Can you work these out from the drawing? Everything is in mm from the part's minimum corner. A direction names the side the tool comes from. Coordinates: 2 decimals unless noted, no trailing zeros. Order: outer loops, then holes, each group sorted by start corner. A loop starts at its lowest first (then second) coordinate and runs counter-clockwise, first axis right, second up. Notation, with made-up numbers: (28, -29) - (47, -29) arc R25 ccw to (47, 0) - close; hole circle Ø9 at (12, -6.75). An arc over 180 degrees is marked (long way). Use a Markdown table: item, result. Add a question column.
(1) I want a section at A-A (x = 3). List the corners of the cut face in (y, z) for me.
(2) For pin 1 Ø2 at (x, y) = (3, 2.2) entering from +Z; pin 2 Ø2.5 at (y, z) = (8.7, 4) entering from -X, each with a flat end and sliding along its axis, tell me the tip position at first contact or that it passes through.
(3) We'd pull the mould along Z, two halves only. Please class the marked faces 3, 4, 5 and 6: pulls with the +Z half, pulls with the -Z half, needs draft (parallel to the pull), parting line crosses it, or undercut.
(4) On a 3-axis mill with a long thin cutter (end or side, diameter ignored), from which of +Z, -Z, +X, -X, +Y, -Y can I reach the whole of each face in a straight line? I mean the marked faces 1 and 2. Say none if no direction works.
(5) I want a section at D-D (z = 6.75). List the corners of the cut face in (x, y) for me, and give its area (3 significant figures).
(6) I want a section at C-C (x = 0.9). List the corners of the cut face in (y, z) for me.
(7) If I drill on L1, parallel to Y at x = 3, z = 6.25; L2, parallel to Z at x = 1.9, y = 42.7; L3, parallel to Y at x = 3, z = 4, over which ranges is the centre line in solid material (lowest first)? Write a range as [from, to].
(8) I want a section at B-B (y = 49.2). List the corners of the cut face in (x, z) for me.
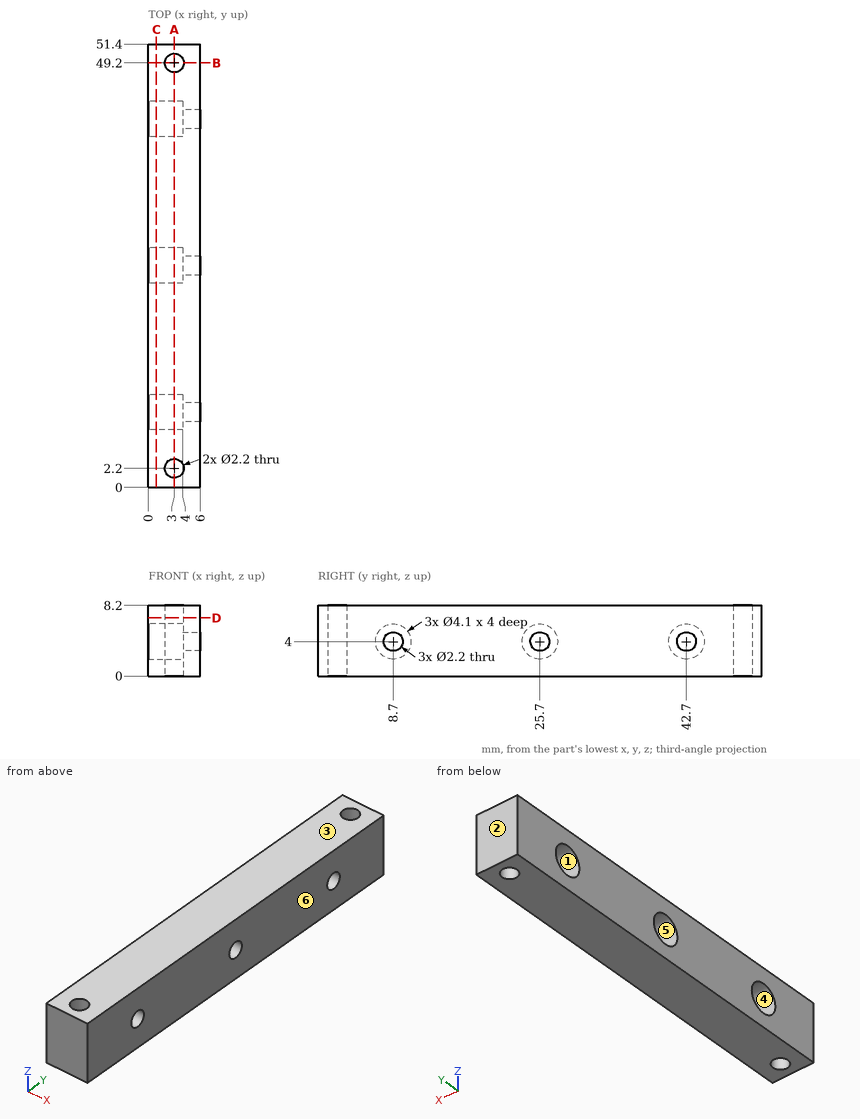
Answers follow:
| question | item | result |
|---|---|---|
| 1 | outline | (0, 0) - (1.1, 0) - (1.1, 8.2) - (0, 8.2) - close; (3.3, 0) - (48.1, 0) - (48.1, 8.2) - (3.3, 8.2) - close; (50.3, 0) - (51.4, 0) - (51.4, 8.2) - (50.3, 8.2) - close; hole circle Ø4.1 at (8.7, 4); hole circle Ø4.1 at (25.7, 4); hole circle Ø4.1 at (42.7, 4) |
| 2 | pin 1 | passes through |
| 2 | pin 2 | stops at x = 4 |
| 3 | face 3 | pulls with the +Z half |
| 3 | face 4 | undercut |
| 3 | face 5 | undercut |
| 3 | face 6 | needs draft |
| 4 | face 1 | -X |
| 4 | face 2 | +Z, -Z, +X, -X, +Y |
| 5 | outline | (0, 0) - (6, 0) - (6, 51.4) - (0, 51.4) - close; hole circle Ø2.2 at (3, 2.2); hole circle Ø2.2 at (3, 49.2) |
| 5 | area | 301 mm² |
| 6 | outline | (0, 0) - (51.4, 0) - (51.4, 8.2) - (0, 8.2) - close; hole circle Ø4.1 at (8.7, 4); hole circle Ø4.1 at (25.7, 4); hole circle Ø4.1 at (42.7, 4) |
| 7 | L1 | y = [0, 1.1], [3.3, 48.1], [50.3, 51.4] |
| 7 | L2 | z = [0, 1.95], [6.05, 8.2] |
| 7 | L3 | y = [0, 1.1], [3.3, 6.65], [10.75, 23.65], [27.75, 40.65], [44.75, 48.1], [50.3, 51.4] |
| 8 | outline | (0, 0) - (1.9, 0) - (1.9, 8.2) - (0, 8.2) - close; (4.1, 0) - (6, 0) - (6, 8.2) - (4.1, 8.2) - close |
